For this review, take the finished solid that the model builds, in its own axes (mm). A direction names the side the tool comes from. Give positions to 0.01 mm unless a question says otherwise; leave off trailing zeros. Loops run counter-clockwise (first coordinate to the right, second up) from the corner with the lowest first, then second, coordinate; pieces in that order, holes last. Notation, with made-up numbers: (-33.75, -30) - (1.25, -30) arc R19 cw to (1.25, -23) - close; hole circle Ø1 at (-28.5, 35.25). An arc over 180 degrees is marked (long way). Put each result on its own line as item: value.
from build123d import *

# Parameters (mm, degrees)
CHAMFER1_SIZE = 0.5715


with BuildPart() as part:
    # Sweep2: sweep along a path in Sketch3
    with BuildLine(Plane.XY) as sweep2_path:
        Line((1.016, -0.0254), (-19.05, -0.0254))
        ThreePointArc((-19.05, -0.0254), (-20.559965377, -0.267702741), (-21.918306738, -0.97028))
        ThreePointArc((-21.918306738, -0.97028), (-23.841883423, 0), (-21.918306738, 0.97028))
        ThreePointArc((-21.918306738, 0.97028), (-20.559965377, 0.267702741), (-19.05, 0.0254))
        Line((-19.05, 0.0254), (0, 0.0254))
    # Sketch4 → Sweep2 (sweep)
    with BuildSketch(Plane(origin=(0, 0, 0), x_dir=(0, 0, -1), z_dir=(1, 0, 0))):
        with BuildLine():
            Line((-1.143, 0.0254), (1.143, 0.0254))
            ThreePointArc((1.143, 0.0254), (0, 1.143), (-1.143, 0.0254))
        make_face()
    sweep(path=sweep2_path.line)

    # Chamfer1
    chamfer1_edges = [part.edges().sort_by_distance(p)[0] for p in [
        (0, 1.143, 0),
        (1.016, -1.143, 0),
    ]]
    chamfer(chamfer1_edges, length=CHAMFER1_SIZE)


solid = part.part
1) Draft analysis for pull direction Y (two halves, no side actions). For faces 3 (the face through (-20.58, 0.274, -0.016)), 4 (the face through (-9.681, 1.143, -0.025)), 5 (the face through (-9.439, -1.143, -0.025)), state which applies: pulls with the +Y half, pulls with the -Y half, needs draft (parallel to the pull), parting line crosses it, or undercut.
Geometry check:
face 3: undercut
face 4: pulls with the +Y half
face 5: pulls with the -Y half
2) Wall thickness on line 1 (Y direction, x = -23.5, z = -0.1); line 2 (Y direction, x = -19.75, z = -0.5); line 3 (X direction, y = -0.55, z = -0.8): over which ranges is each line inside the solid? List them lowest first.
Geometry check:
line 1: y = -2.15 to -0.84, 0.84 to 2.15
line 2: y = -1.09 to -0.08, 0.08 to 1.09
line 3: x = -24.56 to -23.71, -21.24 to 0.62
3) For faces 1 (the face through (-0.155, 0.726, -0.016)), 2 (the face through (-20.54, -0.26, -0.02)), list the 3-axis set-ups (+Z, -Z, +X, -X, +Y, -Y) from which the entire face can be reached by the end or side of a thin tool; tool diameter is ignored.
Geometry check:
face 1: +X, +Y
face 2: +Z, -Z
4) Take a section at A-A on x = -4.5. State the section outline as (y, z) points, and give its area (3 significant figures).
Geometry check:
outline: (-0.03, -1.14) - (-0.03, 1.14) arc R1.14 ccw to start; (0.03, -1.14) arc R1.14 ccw to (0.03, 1.14) - close
area: 3.99 mm²
5) Insertion check: pin 1 Ø1 at (y, z) = (0.5, 0) entering from -X; pin 2 Ø0.6 at (y, z) = (0.5, 0) entering from +X. Each pin has a flat end and moves straight along its axis. Give the tip position at first contact, or say it passes through.
Geometry check:
pin 1: stops at x = -24.96
pin 2: stops at x = 0
